from build123d import *

# Parameters (mm, degrees)
SKETCH1_W           = 400
SKETCH1_H           = 270
BOSS_EXTRUDE1_DEPTH = 70
FILLET1_R           = 7.5
SKETCH3_W           = 120
SKETCH3_H           = 120
CUT_EXTRUDE1_DEPTH  = 63
SKETCH5_W           = 120
SKETCH5_H           = 12
CUT_EXTRUDE2_DEPTH  = 153
SKETCH6_W           = 120
SKETCH6_H           = 12
CUT_EXTRUDE3_DEPTH  = 153
CUT_EXTRUDE4_REACH  = 255.281
SKETCH7_W           = 18
SKETCH7_H           = 12


with BuildPart() as part:
    # Sketch1 → Boss-Extrude1 (new body)
    with BuildSketch(Plane(origin=(0, 0, 0), x_dir=(1, 0, 0), z_dir=(0, 1, 0))):
        Rectangle(SKETCH1_W, SKETCH1_H)
    extrude(amount=BOSS_EXTRUDE1_DEPTH)

    # Fillet1
    fillet1_edges = [part.edges().sort_by_distance(p)[0] for p in [
        (-200, 35, -135),
        (200, 35, -135),
        (200, 35, 135),
        (-200, 35, 135),
    ]]
    fillet(fillet1_edges, radius=FILLET1_R)

    # Sketch3 → Cut-Extrude1 (cut)
    with BuildSketch(Plane(origin=(0, 70, 0), x_dir=(1, 0, 0), z_dir=(0, 1, 0))):
        with Locations((0, 63.749469805)):
            Rectangle(SKETCH3_W, SKETCH3_H)
        with Locations((-132.500014476, 63.749478681)):
            Rectangle(SKETCH3_W, SKETCH3_H)
        with Locations((132.500029203, 63.749477903)):
            Rectangle(SKETCH3_W, SKETCH3_H)
        with Locations((132.500029203, -63.749477903)):
            Rectangle(SKETCH3_W, SKETCH3_H)
        with Locations((0, -63.749469805)):
            Rectangle(SKETCH3_W, SKETCH3_H)
        with Locations((-132.500014476, -63.749478681)):
            Rectangle(SKETCH3_W, SKETCH3_H)
    extrude(amount=-CUT_EXTRUDE1_DEPTH, mode=Mode.SUBTRACT)

    # Sketch5 → Cut-Extrude2 (cut)
    with BuildSketch(Plane.ZY.offset(72.500014476)):
        with Locations((-63.749478681, 13)):
            Rectangle(SKETCH5_W, SKETCH5_H)
    extrude(amount=-CUT_EXTRUDE2_DEPTH, mode=Mode.SUBTRACT)

    # Sketch6 → Cut-Extrude3 (cut)
    with BuildSketch(Plane.ZY.offset(72.500014476)):
        with Locations((63.749478681, 13)):
            Rectangle(SKETCH6_W, SKETCH6_H)
    extrude(amount=-CUT_EXTRUDE3_DEPTH, mode=Mode.SUBTRACT)

    # Sketch7 → Cut-Extrude4 (cut, up to next)
    with BuildSketch(Plane.XY.offset(3.749477903), mode=Mode.PRIVATE) as cut_extrude4_sk1:
        with Locations((-51, 13)):
            Rectangle(SKETCH7_W, SKETCH7_H)
    cut_extrude4_tool1 = extrude(cut_extrude4_sk1.sketch, amount=-CUT_EXTRUDE4_REACH, mode=Mode.PRIVATE) & part.part
    # Sketch7 → Cut-Extrude4 (cut, up to next)
    with BuildSketch(Plane.XY.offset(3.749477903), mode=Mode.PRIVATE) as cut_extrude4_sk2:
        with Locations((51, 13)):
            Rectangle(SKETCH7_W, SKETCH7_H)
    cut_extrude4_tool2 = extrude(cut_extrude4_sk2.sketch, amount=-CUT_EXTRUDE4_REACH, mode=Mode.PRIVATE) & part.part
    add(cut_extrude4_tool1.solids().sort_by_distance((-51, 13, 3.749478))[0], mode=Mode.SUBTRACT)
    add(cut_extrude4_tool2.solids().sort_by_distance((51, 13, 3.749478))[0], mode=Mode.SUBTRACT)


solid = part.part
Work out the finished part from the listing and answer in its coordinate system (mm). A direction names the side the tool comes from. Round coordinates to 2 decimals unless told otherwise and drop trailing zeros. Loops run counter-clockwise (first coordinate to the right, second up) from the corner with the lowest first, then second, coordinate; pieces in that order, holes last. Notation, with made-up numbers: (15, -7.5) - (52, -7.5) arc R18 ccw to (52, 14.5) - close; hole circle Ø7 at (-12.5, -14.5). An arc over 180 degrees is marked (long way). One line per item, written item: value.
Q1. Find section A-A on y = 12.5. State how many separate pieces and enclosed holes the cut face has, and give its area (3 significant figures).
Check values:
separate pieces: 2
enclosed holes: 1
area: 15,300 mm2
Q2. For faces 5 (the flat face through (-45, 70, -1)), 6 (the flat face through (72.5, 46, 65)), 7 (the flat face through (51, 19, 0)), determine the directions among +Z, -Z, +X, -X, +Y, -Y from which every point of the face is accessible in a straight line to the end or side of a thin tool.
Check values:
face 5: +Z, -Z, +X, -X, +Y
face 6: +Y
face 7: none
Q3. Find section B-B on z = 8.5. Give the vertices of the cut face in (x, y).
Check values:
outline: (-200, 0) - (200, 0) - (200, 70) - (192.5, 70) - (192.5, 7) - (-192.5, 7) - (-192.5, 70) - (-200, 70) - close; (-72.5, 19) - (-60, 19) - (-60, 70) - (-72.5, 70) - close; (60, 19) - (72.5, 19) - (72.5, 70) - (60, 70) - close
Q4. The mould has two halves that part along X. Classify faces 1 (the flat face through (-200, 35, 2)), 2 (the cylindrical face through (197.861, 35.49, -132.745)), 3 (the flat face through (-3, 35, 135)), 4 (the flat face through (-3, 7, -29)): +X half, -X half, draft (parallel to the pull), parting line (faces both ways), or undercut.
Check values:
face 1: -X half
face 2: +X half
face 3: draft
face 4: undercut
Q5. This flat-tipped pin is pushed along its axis until it touches: pin 1 Ø3 at (x, z) = (51, 93.5) entering from +Y. Where does it stop, or does it pass through?
Check values:
pin 1: y = 7
Q6. Find section D-D on x = 109.5. Give the vertices of the cut face in (y, z), and give its area (3 significant figures).
Check values:
outline: (0, -135) - (70, -135) - (70, -123.75) - (7, -123.75) - (7, -3.75) - (70, -3.75) - (70, 3.75) - (7, 3.75) - (7, 123.75) - (70, 123.75) - (70, 135) - (0, 135) - close
area: 3,780 mm2
Q7. Straight lines are drawn through the part: probe 1 along Z at (x, y) = (112, 61.5); probe 2 along X at (y, z) = (47.5, -115.5); probe 3 along X at (y, z) = (9, 38.5). For each, find the intervals that lie inside material, in ascending order.
Check values:
probe 1: -135 to -123.75, -3.75 to 3.75, 123.75 to 135
probe 2: -200 to -192.5, -72.5 to -60, 60 to 72.5, 192.5 to 200
probe 3: -200 to -192.5, 192.5 to 200
